The figure shows three views and two pictorial views of one solid part (mm, origin at its lowest corner). Answer the questions. Round coordinates to 2 decimals unless told otherwise and drop trailing zeros. Order: outer loops, then holes, each group sorted by start corner. A loop starts at its lowest first (then second) coordinate and runs counter-clockwise, first axis right, second up.
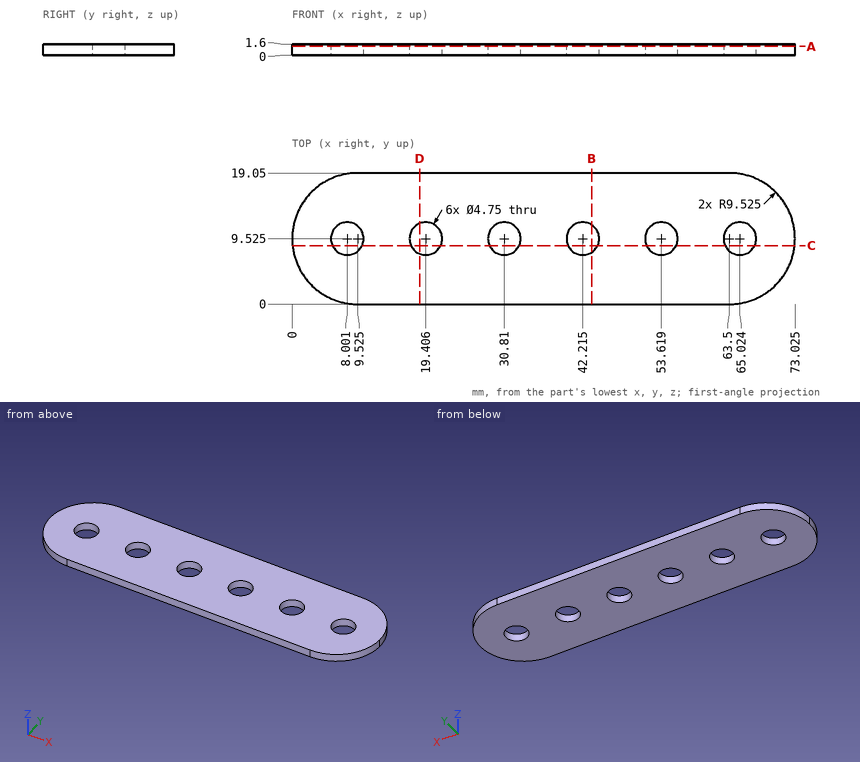
Item 1: Find the intervals of material crossed by line 1 along Y through (x, z) = (42, 1.1); line 2 along Y through (x, z) = (52, 0.2); line 3 along X through (y, z) = (6.5, 0.15), in increasing order.
Item 2: Given pin 1 (5.5 mm diameter, centred on x = 30.81, y = 9.52, fed in from -Z), flat-ended and moving along its own axis, determine where the tip first touches the part or whether it passes through.
Item 3: Find section A-A (z = 1.25). State how many separate pieces and enclosed holes the cut face has, plus the area to 3 significant figures.
Item 4: Find section B-B (x = 43.5). Write down the section's boundary in (y, z), plus the area to 3 significant figures.
Item 5: Find section C-C (y = 8.5). Write down the section's boundary in (x, z) (1 decimal).
Item 6: Find section D-D (x = 18.5). Write down the section's boundary in (y, z).
Model answer:
1. line 1: y = 0 to 7.16, 11.89 to 19.05
1. line 2: y = 0 to 7.79, 11.26 to 19.05
1. line 3: x = 0.49 to 72.53
2. pin 1: stops at z = 0
3. separate pieces: 1
3. enclosed holes: 6
3. area: 1,210 mm2
4. outline: (0, 0) - (7.53, 0) - (7.53, 1.6) - (0, 1.6) - close; (11.52, 0) - (19.05, 0) - (19.05, 1.6) - (11.52, 1.6) - close
4. area: 24.1 mm2
5. outline: (0.1, 0) - (5.9, 0) - (5.9, 1.6) - (0.1, 1.6) - close; (10.1, 0) - (17.3, 0) - (17.3, 1.6) - (10.1, 1.6) - close; (21.5, 0) - (28.7, 0) - (28.7, 1.6) - (21.5, 1.6) - close; (33, 0) - (40.1, 0) - (40.1, 1.6) - (33, 1.6) - close; (44.4, 0) - (51.5, 0) - (51.5, 1.6) - (44.4, 1.6) - close; (55.8, 0) - (62.9, 0) - (62.9, 1.6) - (55.8, 1.6) - close; (67.2, 0) - (73, 0) - (73, 1.6) - (67.2, 1.6) - close
6. outline: (0, 0) - (7.33, 0) - (7.33, 1.6) - (0, 1.6) - close; (11.72, 0) - (19.05, 0) - (19.05, 1.6) - (11.72, 1.6) - close
